```python
from build123d import *

# Parameters (mm, degrees)
SKETCH1_R                = 3.5
SKETCH1_R_2              = 1.75
BOSS_EXTRUDE1_DEPTH      = 10
SKETCH3_R                = 3.5
BOSS_EXTRUDE2_DEPTH      = 1
BOSS_EXTRUDE3_DEPTH      = 1
BOSS_EXTRUDE3_DEPTH_BACK = 1


with BuildPart() as part:
    # Sketch1 → Boss-Extrude1 (new body)
    with BuildSketch(Plane(origin=(0, 0, 0), x_dir=(1, 0, 0), z_dir=(0, 1, 0))):
        Circle(SKETCH1_R)
        Circle(SKETCH1_R_2, mode=Mode.SUBTRACT)
    extrude(amount=BOSS_EXTRUDE1_DEPTH)

    # Sketch3 → Boss-Extrude2 (add)
    with BuildSketch(Plane(origin=(0, 10, 0), x_dir=(1, 0, 0), z_dir=(0, 1, 0))):
        Circle(SKETCH3_R)
    extrude(amount=BOSS_EXTRUDE2_DEPTH)

    # Sketch2 → Boss-Extrude3 (add, two sides)
    with BuildSketch(Plane.XY) as boss_extrude3_sk:
        with BuildLine():
            Line((-4.811497646, 15.640040293), (-3.5, 11))
            Line((-3.5, 11), (3.5, 11))
            Line((3.5, 11), (4.811497646, 15.640040293))
            ThreePointArc((4.811497646, 15.640040293), (0, 22), (-4.811497646, 15.640040293))
        make_face()
    extrude(amount=BOSS_EXTRUDE3_DEPTH)
    extrude(boss_extrude3_sk.sketch, amount=-BOSS_EXTRUDE3_DEPTH_BACK)

    # Sketch4 → Cut-Revolve1 (revolve, cut)
    with BuildSketch(Plane.XY):
        with BuildLine():
            Line((0, 20), (0, 14))
            ThreePointArc((0, 14), (3, 17), (0, 20))
        make_face()
    revolve(axis=Axis((0, 22, 0), (0, -1, 0)), mode=Mode.SUBTRACT)


solid = part.part
```
Input: part model. Units: mm. Frame: model coordinates. A direction names the side the tool comes from. Coordinates: 2 decimals unless noted, no trailing zeros. Loops run counter-clockwise (first coordinate to the right, second up) from the corner with the lowest first, then second, coordinate; pieces in that order, holes last. Notation, with made-up numbers: M 37.25,-40 L 66.25,-40 A30 cw 66.25,-9 Z; hole C 4.5,89.25 d7. An arc over 180 degrees is marked long. Use a Markdown table: item, result. Add a question column.
1) Section A-A, the plane x = 0. Return the cut outline in (y, z).
2) Line query: L1, parallel to X at y = 3.5, z = 0; L2, parallel to Z at x = 3, y = 18.5. Output: solid intervals per line, ascending. Write a range as from..to.
3) Draft query along X for faces 1 (the cylindrical face through (1.617, 4.93, 0.67)), 2 (the flat face through (0, 11, -2)), 3 (the cylindrical face through (3.233, 5.423, 1.341)). Return one class per face: +X half, -X half, draft (parallel to the pull), parting line (faces both ways), or undercut.
4) Set-up query: faces 4 (the flat face through (0, 11, 2)), 5 (the flat face through (0, 14, -1)), 6 (the flat face through (0, 10, 0)). Return all of +Z, -Z, +X, -X, +Y, -Y with unobstructed straight access to the full face (end or side cutting, diameter ignored); none if empty.
5) Pin query (flat end, axial travel): P1, Ø3, axis at y = 8, z = -1, coming from the -X side; P2, Ø1, axis at x = 0.5, z = 0.5, coming from the -Y side; P3, Ø1, axis at y = 8, z = -1, coming from the +X side. Return the tip coordinate at first contact, or that it passes through.
6) Section C-C, the plane y = 17. Return the cut outline in (x, z).
7) Section B-B, the plane y = 2.5. Return the cut outline in (x, z).
Answer below:
| question | item | result |
|---|---|---|
| 1 | outline | M 0,-3.5 L 11,-3.5 L 11,-1 L 14.17,-1 A3 cw 14.17,1 L 11,1 L 11,3.5 L 0,3.5 L 0,1.75 L 10,1.75 L 10,-1.75 L 0,-1.75 Z; M 19.83,-1 L 22,-1 L 22,1 L 19.83,1 A3 cw Z |
| 2 | L1 | -3.5..-1.75, 1.75..3.5 |
| 2 | L2 | -1..1 |
| 3 | face 1 | undercut |
| 3 | face 2 | draft |
| 3 | face 3 | parting line |
| 4 | face 4 | +Z, +X, -X, +Y |
| 4 | face 5 | -Z, +X, -X, +Y |
| 4 | face 6 | -Y |
| 5 | P1 | x = -3.5 |
| 5 | P2 | y = 10 |
| 5 | P3 | x = 3.46 |
| 6 | outline | M -5,-1 L -2.83,-1 A3 cw -2.83,1 L -5,1 Z; M 2.83,-1 L 5,-1 L 5,1 L 2.83,1 A3 cw Z |
| 7 | outline | C 0,0 d7; hole C 0,0 d3.5 |
